For this review, use the dimensioned drawing (mm, ordinates from the lowest corner) and the shaded views. A direction names the side the tool comes from. Round coordinates to 2 decimals unless told otherwise and drop trailing zeros. Loops run counter-clockwise (first coordinate to the right, second up) from the corner with the lowest first, then second, coordinate; pieces in that order, holes last. Notation, with made-up numbers: (56, 76) - (90, 76) arc R32 ccw to (90, 114) - close; hole circle Ø3 at (52, 10.5). An arc over 180 degrees is marked (long way). Answer as CSV lines item,"result". Start each with the question number.
(1) For P1, Ø1.5, axis at x = 2.5, z = 2.5, coming from the +Y side; P2, Ø0.9, axis at x = 1.5, z = 6, coming from the +Y side, all flat-tipped, find the tip position at first contact; note any pin that passes through.
(2) Consider section A-A (y = 6). Give the boundary of the cut face in (x, z).
(3) For the marked faces 4 and 5, list the 3-axis set-ups (+Z, -Z, +X, -X, +Y, -Y) from which the entire face can be reached by the end or side of a thin tool; tool diameter is ignored.
(4) Mouldability with a two-part tool opening along Y and no side actions: class the marked faces 1, 2 and 3 as released by +Y, released by -Y, zero draft, split by the parting line, or undercut.
(5) Consider section C-C (x = 2.5). Give the boundary of the cut face in (y, z).
(6) Consider section B-B (z = 6). Give the boundary of the cut face in (x, y).
(7) Wall thickness on L1, parallel to Z at x = 1.65, y = 1; L2, parallel to Y at x = 1.4, z = 8.5; L3, parallel to Y at x = 2.2, z = 4: over which ranges is each line inside the solid? List them lowest first.
(8) Consider section D-D (z = 4.75). Give the boundary of the cut face in (x, y), and give its area (3 significant figures).
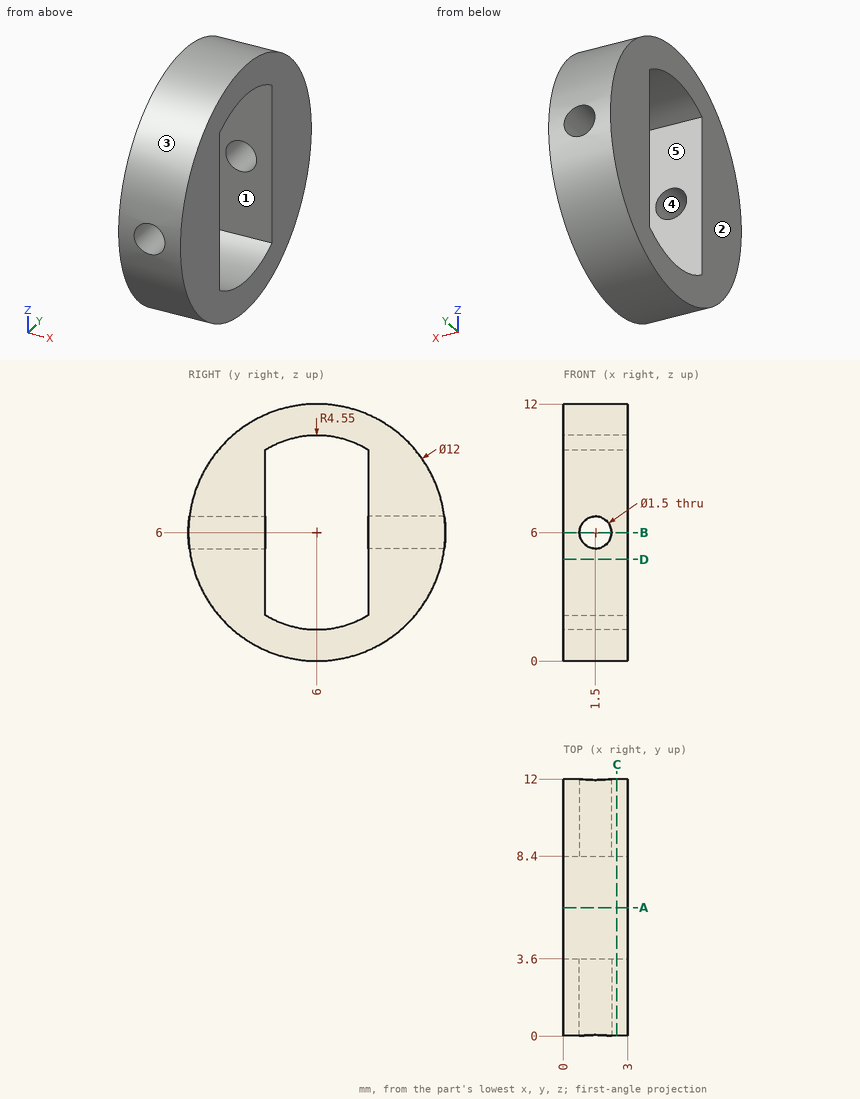
Determined:
1,P1,"stops at y = 11.33"
1,P2,"passes through"
2,outline,"(0, 0) - (3, 0) - (3, 1.45) - (0, 1.45) - close; (0, 10.55) - (3, 10.55) - (3, 12) - (0, 12) - close"
3,face 4,"+Y, -Y"
3,face 5,"+X, -X"
4,face 1,"undercut"
4,face 2,"zero draft"
4,face 3,"split by the parting line"
5,outline,"circle Ø12 at (6, 6); hole (3.6, 2.13) arc R4.55 ccw to (8.4, 2.13) - (8.4, 9.87) arc R4.55 ccw to (3.6, 9.87) - close"
6,outline,"(0, 0) - (0.75, 0) - (0.75, 3.6) - (0, 3.6) - close; (0, 8.4) - (0.75, 8.4) - (0.75, 12) - (0, 12) - close; (2.25, 0) - (3, 0) - (3, 3.6) - (2.25, 3.6) - close; (2.25, 8.4) - (3, 8.4) - (3, 12) - (2.25, 12) - close"
7,L1,"z = 2.68 to 5.27, 6.73 to 9.32"
7,L2,"y = 0.55 to 3.6, 8.4 to 11.45"
7,L3,"y = 0.34 to 3.6, 8.4 to 11.66"
8,outline,"(0, 0.13) - (3, 0.13) - (3, 3.6) - (0, 3.6) - close; (0, 8.4) - (3, 8.4) - (3, 11.87) - (0, 11.87) - close"
8,area,"20.8 mm^2"
